The model under review builds one solid part; all positions refer to its coordinate system, in mm. A direction names the side the tool comes from. Coordinates: 2 decimals unless noted, no trailing zeros. Write each loop counter-clockwise with the first axis right and the second up, starting at its lowest first coordinate (ties: lowest second). Pieces come first, ordered by that corner, then holes.
1) For line 1 (X direction, y = 48, z = 59); line 2 (X direction, y = 44, z = 49); line 3 (Y direction, x = 31, z = 63.5), list the stretches that pass through material, from the lowest coordinate up.
2) Add section A-A, the plane y = 30. State the section outline as (x, z) points, then the cut area to 3 significant figures.
3) Add section D-D, the plane y = 11. State the section outline as (x, z) points.
4) Mouldability with a two-part tool opening along X and no side actions: class faces 4 (the flat face through (42, 41, 24)), 5 (the flat face through (21, 20, 20)), 6 (the cylindrical face through (20.84, 46.2, 50.24)) as released by +X, released by -X, zero draft, split by the parting line, or undercut.
5) Add section B-B, the plane z = 7.5. State the section outline as (x, y) points.
6) For P1, Ø2, axis at x = 38, z = 59, coming from the -Y side; P2, Ø2, axis at x = 21, z = 49, coming from the +Y side; P3, Ø1.5, axis at x = 4, z = 59, coming from the +Y side, all flat-tipped, find the tip position at first contact; note any pin that passes through.
7) Add section C-C, the plane x = 7. State the section outline as (y, z) points.
8) Machinability: for faces 1 (the cylindrical face through (3.84, 46.2, 60.24)), 2 (the flat face through (21, 40, 54)), 3 (the flat face through (21, 25, 0)), which of the approach directions +Z, -Z, +X, -X, +Y, -Y give a long, thin tool a straight path to every point of the face, cutting with its end or side? Answer none if there is none.
from build123d import *

# Parameters (mm, degrees)
SKETCH_1_W             = 42
SKETCH_1_H             = 50
EXTRUDE_1_DEPTH        = 87
SKETCH_2_W             = 67
SKETCH_2_H             = 40
CUT_EXTRUDE_1_DEPTH    = 109.779593675
SKETCH_3_R             = 2.75
CUT_EXTRUDE_2_DEPTH    = 94.55746897
HOLE_WIZARD_M3_1_D     = 2.5
HOLE_WIZARD_M3_1_DEPTH = 7.5
HOLE_WIZARD_M3_1_TIP   = 0.751075774


with BuildPart() as part:
    # 草图1 → 凸台-拉伸1 (new body)
    with BuildSketch(Plane.XY):
        with Locations((21, 25)):
            Rectangle(SKETCH_1_W, SKETCH_1_H)
    extrude(amount=EXTRUDE_1_DEPTH)

    # 草图2 → 切除-拉伸1 (cut, through all)
    with BuildSketch(Plane(origin=(42, 0, 0), x_dir=(0, 0, -1), z_dir=(1, 0, 0))):
        with Locations((-53.5, 20)):
            Rectangle(SKETCH_2_W, SKETCH_2_H)
    extrude(amount=-CUT_EXTRUDE_1_DEPTH, mode=Mode.SUBTRACT)

    # 草图3 → 切除-拉伸2 (cut, through all)
    with BuildSketch(Plane.XY.offset(20)):
        with Locations((7, 30)):
            Circle(SKETCH_3_R)
        with Locations((7, 10)):
            Circle(SKETCH_3_R)
        with Locations(Location((35, 10, 0), (0, 0, 180))):
            Circle(SKETCH_3_R)
        with Locations(Location((35, 30, 0), (0, 0, 180))):
            Circle(SKETCH_3_R)
    extrude(amount=-CUT_EXTRUDE_2_DEPTH, mode=Mode.SUBTRACT)

    # M3 螺纹孔1
    with Locations(Plane(origin=(0, 50, 0), x_dir=(-1, 0, 0), z_dir=(0, 1, 0))):
        with Locations((-4, 59), (-21, 49), (-38, 59), (-21, 69)):
            Hole(HOLE_WIZARD_M3_1_D / 2, depth=HOLE_WIZARD_M3_1_DEPTH)
            with Locations((0, 0, -(HOLE_WIZARD_M3_1_DEPTH + HOLE_WIZARD_M3_1_TIP / 2))):  # 118° drill point
                Cone(0, HOLE_WIZARD_M3_1_D / 2, HOLE_WIZARD_M3_1_TIP, mode=Mode.SUBTRACT)


solid = part.part
Geometry results:
1. line 1: x = 0 to 2.75, 5.25 to 36.75, 39.25 to 42
1. line 2: x = 0 to 19.75, 22.25 to 42
1. line 3: y = 40 to 50
2. outline: (0, 0) - (4.25, 0) - (4.25, 20) - (0, 20) - close; (9.75, 0) - (32.25, 0) - (32.25, 20) - (9.75, 20) - close; (37.75, 0) - (42, 0) - (42, 20) - (37.75, 20) - close
2. area: 620 mm2
3. outline: (0, 0) - (4.44, 0) - (4.44, 20) - (0, 20) - close; (9.56, 0) - (32.44, 0) - (32.44, 20) - (9.56, 20) - close; (37.56, 0) - (42, 0) - (42, 20) - (37.56, 20) - close
4. face 4: released by +X
4. face 5: zero draft
4. face 6: undercut
5. outline: (0, 0) - (42, 0) - (42, 50) - (0, 50) - close; hole circle Ø5.5 at (7, 10); hole circle Ø5.5 at (7, 30); hole circle Ø5.5 at (35, 10); hole circle Ø5.5 at (35, 30)
6. P1: stops at y = 40
6. P2: stops at y = 42.35
6. P3: stops at y = 42.2
7. outline: (0, 0) - (7.25, 0) - (7.25, 20) - (0, 20) - close; (12.75, 0) - (27.25, 0) - (27.25, 20) - (12.75, 20) - close; (32.75, 0) - (50, 0) - (50, 87) - (40, 87) - (40, 20) - (32.75, 20) - close
8. face 1: +Y
8. face 2: +Z, +X, -X, -Y
8. face 3: -Z, +X, -X, +Y, -Y
